For this review, take the finished solid that the model builds, in its own axes (mm). Face numbers are marked on the shaded views. Round coordinates to 2 decimals unless told otherwise and drop trailing zeros. Loops run counter-clockwise (first coordinate to the right, second up) from the corner with the lowest first, then second, coordinate; pieces in that order, holes last.
```python
from build123d import *

# Parameters (mm, degrees)
SKETCH1_R           = 3.375
BOSS_EXTRUDE1_DEPTH = 1.65
SKETCH2_R           = 1.5
BOSS_EXTRUDE2_DEPTH = 18.35
CHAMFER1_SIZE       = 0.3
CUT_EXTRUDE1_DEPTH  = 2
CHAMFER2_SIZE       = 1.65


with BuildPart() as part:
    # Sketch1 → Boss-Extrude1 (new body)
    with BuildSketch(Plane.XY):
        Circle(SKETCH1_R)
    extrude(amount=BOSS_EXTRUDE1_DEPTH)

    # Sketch2 → Boss-Extrude2 (add)
    with BuildSketch(Plane(origin=(0, 0, 0), x_dir=(-1, 0, 0), z_dir=(0, 0, -1))):
        with Locations(Location((0, 0, 0), (0, 0, 180))):
            Circle(SKETCH2_R)
    extrude(amount=BOSS_EXTRUDE2_DEPTH)

    # Chamfer1
    chamfer1_edges = [part.edges().sort_by_distance(p)[0] for p in [
        (-1.5, 0, -18.35),
    ]]
    chamfer(chamfer1_edges, length=CHAMFER1_SIZE)

    # Sketch3 → Cut-Extrude1 (cut)
    with BuildSketch(Plane.XY.offset(1.65)):
        Polygon((0, 1.154700538), (-1, 0.577350269), (-1, -0.577350269), (0, -1.154700538), (1, -0.577350269), (1, 0.577350269), align=None)
    extrude(amount=-CUT_EXTRUDE1_DEPTH, mode=Mode.SUBTRACT)

    # Chamfer2
    chamfer2_edges = [part.edges().sort_by_distance(p)[0] for p in [
        (-3.375, 0, 0),
    ]]
    chamfer(chamfer2_edges, length=CHAMFER2_SIZE - 0.0001)  # a hair under: the kernel refuses the full size


solid = part.part
```
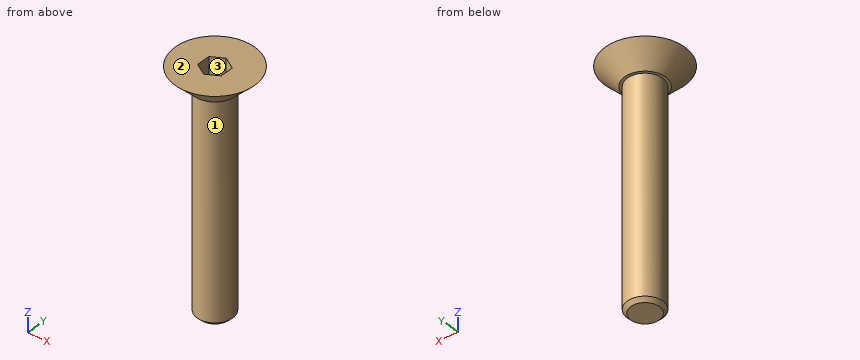
(1) The part is to be moulded in two halves that separate along X. For the marked faces 1, 2 and 3, say which applies: pulls with the +X half, pulls with the -X half, needs draft (parallel to the pull), parting line crosses it, or undercut.
(2) Insertion check: pin 1 Ø4 at (y, z) = (-0.5, -14) entering from +X; pin 2 Ø1 at (x, z) = (1.5, -2.5) entering from -Y. Each pin has a flat end and moves straight along its axis. Give the tip position at first contact, or say it passes through.
(3) Add section B-B (z = -11.5). Give the boundary of the cut face in (x, y), plus the area to 3 significant figures.
(4) For L1, parallel to Y at x = 0, z = -15.25; L2, parallel to Y at x = -0.75, z = -1.75; L3, parallel to Z at x = 3, y = 1, list the stretches that pass through material, from the lowest coordinate up.
Outcome:
1. face 1: parting line crosses it
1. face 2: needs draft
1. face 3: undercut
2. pin 1: stops at x = 1.5
2. pin 2: stops at y = -1.12
3. outline: circle Ø3 at (0, 0)
3. area: 7.07 mm2
4. L1: y = -1.5 to 1.5
4. L2: y = -1.3 to 1.3
4. L3: z = 1.44 to 1.65
